For this review, take the finished solid that the model builds, in its own axes (mm). A direction names the side the tool comes from. Coordinates: 2 decimals unless noted, no trailing zeros. One line per item, written item: value. Start each with the question number.
1) For probe 1 along X at (y, z) = (56.5, 1.05); probe 2 along Y at (x, z) = (26, 2.05); probe 3 along Y at (x, z) = (-141.5, 0.25), list the stretches that pass through material, from the lowest coordinate up. Write a range as from..to.
2) Machinability: for faces 1 (the flat face through (-1, -13, 3.175)), 2 (the cylindrical face through (14.35, 78.53, 1.61)), which of the approach directions +Z, -Z, +X, -X, +Y, -Y give a long, thin tool a straight path to every point of the face, cutting with its end or side? Answer none if there is none.
3) For pin 1 Ø1.5 at (x, y) = (138, 114.5) entering from -Z; pin 2 Ø4.5 at (x, y) = (-169.1, 54.94) entering from -Z (3 decimals), all flat-tipped, find the tip position at first contact; note any pin that passes through.
4) Mouldability with a two-part tool opening along Y and no side actions: class faces 3 (the cylindrical face through (-151.17, -115.92, 1.57)), 4 (the cylindrical face through (105.329, 143.243, 1.565)), 5 (the flat face through (-1, -13, 0)) as released by +Y, released by -Y, zero draft, split by the parting line, or undercut.
from build123d import *

# Parameters (mm, degrees)
SKETCH1_R           = 190.5
SKETCH1_R_2         = 12.7
SKETCH1_R_3         = 2.9
SKETCH1_R_4         = 2.032
BOSS_EXTRUDE3_DEPTH = 3.175
FILLET1_R           = 12.7
FILLET2_R           = 12.7
FILLET3_R           = 12.7


with BuildPart() as part:
    # Sketch1 → Boss-Extrude3 (new body)
    with BuildSketch(Plane.XY):
        Circle(SKETCH1_R)
        Circle(SKETCH1_R_2, mode=Mode.SUBTRACT)
        with Locations((-36.235253271, 11.773547486)):
            Circle(SKETCH1_R_3, mode=Mode.SUBTRACT)
        with Locations((-22.394618112, -30.823547486)):
            Circle(SKETCH1_R_3, mode=Mode.SUBTRACT)
        with Locations((22.394618112, -30.823547486)):
            Circle(SKETCH1_R_3, mode=Mode.SUBTRACT)
        with Locations((36.235253271, 11.773547486)):
            Circle(SKETCH1_R_3, mode=Mode.SUBTRACT)
        with Locations((0, 38.1)):
            Circle(SKETCH1_R_3, mode=Mode.SUBTRACT)
        with Locations((-169.097848597, 54.9432216)):
            Circle(SKETCH1_R_3, mode=Mode.SUBTRACT)
        with Locations((0, 177.8)):
            Circle(SKETCH1_R_3, mode=Mode.SUBTRACT)
        with Locations((169.097848597, 54.9432216)):
            Circle(SKETCH1_R_3, mode=Mode.SUBTRACT)
        with Locations((104.508217858, -143.8432216)):
            Circle(SKETCH1_R_3, mode=Mode.SUBTRACT)
        with Locations((-104.508217858, -143.8432216)):
            Circle(SKETCH1_R_3, mode=Mode.SUBTRACT)
        with Locations((-20.677222541, 11.938)):
            Circle(SKETCH1_R_4, mode=Mode.SUBTRACT)
        with Locations((0, 23.876)):
            Circle(SKETCH1_R_4, mode=Mode.SUBTRACT)
        with Locations((20.677222541, 11.938)):
            Circle(SKETCH1_R_4, mode=Mode.SUBTRACT)
        with Locations((20.677222541, -11.938)):
            Circle(SKETCH1_R_4, mode=Mode.SUBTRACT)
        with Locations((0, -23.876)):
            Circle(SKETCH1_R_4, mode=Mode.SUBTRACT)
        with Locations((-20.677222541, -11.938)):
            Circle(SKETCH1_R_4, mode=Mode.SUBTRACT)
        with BuildLine():
            Line((25.335121222, 175.985714286), (10.857909095, 75.42244898))
            ThreePointArc((10.857909095, 75.42244898), (44.789236225, 61.647094971), (68.375733143, 33.63330369))
            Line((68.375733143, 33.63330369), (159.543377334, 78.477708611))
            ThreePointArc((159.543377334, 78.477708611), (104.508217858, 143.8432216), (25.335121222, 175.985714286))
        make_face(mode=Mode.SUBTRACT)
        with BuildLine():
            Line((-25.4, 175.976362049), (-10.885714286, 75.418440878))
            ThreePointArc((-10.885714286, 75.418440878), (-44.800599154, 61.63883772), (-68.375733143, 33.63330369))
            Line((-68.375733143, 33.63330369), (-159.543377334, 78.477708611))
            ThreePointArc((-159.543377334, 78.477708611), (-104.53473136, 143.823954679), (-25.4, 175.976362049))
        make_face(mode=Mode.SUBTRACT)
        with BuildLine():
            Line((75.086290011, 12.980333294), (175.201343359, 30.287444352))
            ThreePointArc((175.201343359, 30.287444352), (169.097848597, -54.9432216), (123.938351095, -127.483823005))
            Line((123.938351095, -127.483823005), (53.116436183, -54.635924145))
            ThreePointArc((53.116436183, -54.635924145), (72.470506542, -23.547094971), (75.086290011, 12.980333294))
        make_face(mode=Mode.SUBTRACT)
        with BuildLine():
            Line((35.547970221, -67.400161819), (82.945263848, -157.267044244))
            ThreePointArc((82.945263848, -157.267044244), (0, -177.8), (-82.945263848, -157.267044244))
            Line((-82.945263848, -157.267044244), (-35.547970221, -67.400161819))
            ThreePointArc((-35.547970221, -67.400161819), (0, -76.2), (35.547970221, -67.400161819))
        make_face(mode=Mode.SUBTRACT)
        with BuildLine():
            Line((-175.201343359, 30.287444352), (-75.086290011, 12.980333294))
            ThreePointArc((-75.086290011, 12.980333294), (-72.470506542, -23.547094971), (-53.116436183, -54.635924145))
            Line((-53.116436183, -54.635924145), (-123.938351095, -127.483823005))
            ThreePointArc((-123.938351095, -127.483823005), (-169.097848597, -54.9432216), (-175.201343359, 30.287444352))
        make_face(mode=Mode.SUBTRACT)
    extrude(amount=BOSS_EXTRUDE3_DEPTH)

    # Fillet1
    fillet1_edges = [part.edges().sort_by_distance(p)[0] for p in [
        (-175.201343359, 30.287444352, 1.5875),
    ]]
    fillet(fillet1_edges, radius=FILLET1_R)

    # Fillet2
    fillet2_edges = [part.edges().sort_by_distance(p)[0] for p in [
        (-25.4, 175.976362049, 1.5875),
        (-159.543377334, 78.477708611, 1.5875),
        (-68.375733143, 33.63330369, 1.5875),
        (-10.885714286, 75.418440878, 1.5875),
        (75.086290011, 12.980333294, 1.5875),
        (53.116436183, -54.635924145, 1.5875),
        (123.938351095, -127.483823005, 1.5875),
        (175.201343359, 30.287444352, 1.5875),
        (35.547970221, -67.400161819, 1.5875),
        (10.857909095, 75.42244898, 1.5875),
        (68.375733143, 33.63330369, 1.5875),
        (159.543377334, 78.477708611, 1.5875),
        (25.335121222, 175.985714286, 1.5875),
    ]]
    fillet(fillet2_edges, radius=FILLET2_R)

    # Fillet3
    fillet3_edges = [part.edges().sort_by_distance(p)[0] for p in [
        (-35.547970221, -67.400161819, 1.5875),
        (-82.945263848, -157.267044244, 1.5875),
        (82.945263848, -157.267044244, 1.5875),
        (-123.938351095, -127.483823005, 1.5875),
        (-53.116436183, -54.635924145, 1.5875),
        (-75.086290011, 12.980333294, 1.5875),
    ]]
    fillet(fillet3_edges, radius=FILLET3_R)


solid = part.part
Numbers:
1. probe 1: -181.93..-171.54, -166.65..-114.86, -51.13..51.13, 114.86..166.65, 171.54..181.93
1. probe 2: -188.72..-175.89, -71.64..71.63, 168.92..188.72
1. probe 3: -127.55..-107.66, 24.46..69.6, 107.66..127.55
2. face 1: +Z, +X, -X, +Y, -Y
2. face 2: +Z, -Z
3. pin 1: z = 0
3. pin 2: through
4. face 3: split by the parting line
4. face 4: undercut
4. face 5: zero draft
